The listing builds one solid part. Answer for the finished solid, in the listing's coordinates (mm). A direction names the side the tool comes from. Give positions to 0.01 mm unless a question says otherwise; leave off trailing zeros. Order: outer loops, then holes, each group sorted by start corner. A loop starts at its lowest first (then second) coordinate and runs counter-clockwise, first axis right, second up. Notation, with made-up numbers: (-28.75, 53.5) - (15.25, 53.5) arc R20 ccw to (15.25, 80.5) - close; hole circle Ø1 at (89.5, 65). An arc over 180 degrees is marked (long way). Use a Markdown table: item, result. Add a question column.
1) Flat-ended cylindrical pins translate along their axes: pin 1 (9 mm diameter, centred on x = -1, z = 0, fed in from +Y); pin 2 (5 mm diameter, centred on x = -12, z = 4.5, fed in from +Y); pin 3 (3 mm diameter, centred on y = -3.5, z = -6, fed in from -X). Find the tip coordinate at first contact, or state that the pin passes through.
2) For faces 4 (the face through (0, -8, 27.5)), 5 (the face through (0, -6, 21.5)), 6 (the face through (5, -4.6, 23.1)), 7 (the face through (0, -12, 25)), 8 (the face through (0, 4, -29.5)), determine the directions among +Z, -Z, +X, -X, +Y, -Y from which every point of the face is accessible in a straight line to the end or side of a thin tool.
3) The mould has two halves that part along Z. Classify faces 1 (the face through (-3.905, 2.986, -0.867)), 2 (the face through (0.07, -1.141, -8.703)), 3 (the face through (-16, 6, 0)): released by +Z, released by -Z, zero draft, split by the parting line, or undercut.
4) Find section B-B, the plane x = 0. State how many separate pieces and enclosed holes the cut face has, plus the area to 3 significant figures.
5) Straight lines are drawn through the part: line 1 (Y direction, x = -0.25, z = -4.5); line 2 (X direction, y = 4.5, z = 19.5); line 3 (Y direction, x = -9, z = -19). For each, find the intervals that lie inside material, in ascending order.
6) Find section D-D, the plane y = -9. Determine the outline of the cut face in (x, z).
7) Find section C-C, the plane z = 11.5. Determine the outline of the cut face in (x, y).
8) Find section A-A, the plane y = -6. Determine the outline of the cut face in (x, z), plus the area to 3 significant figures.
from build123d import *

# Parameters (mm, degrees)
SKETCH1_W           = 35
SKETCH1_H           = 63
BOSS_EXTRUDE1_DEPTH = 2
SKETCH2_W           = 10
SKETCH2_H           = 6
BOSS_EXTRUDE2_DEPTH = 12
SKETCH3_R           = 1.7
CUT_EXTRUDE1_DEPTH  = 10
FILLET1_R           = 4
SKETCH4_W           = 35
SKETCH4_H           = 63
SKETCH4_W_2         = 31
SKETCH4_H_2         = 59
BOSS_EXTRUDE4_DEPTH = 4
SKETCH5_R           = 4
BOSS_EXTRUDE5_DEPTH = 2


with BuildPart() as part:
    # Sketch1 → Boss-Extrude1 (new body)
    with BuildSketch(Plane(origin=(0, 0, 0), x_dir=(1, 0, 0), z_dir=(0, 1, 0))):
        Rectangle(SKETCH1_W, SKETCH1_H)
    extrude(amount=BOSS_EXTRUDE1_DEPTH)

    # Sketch2 → Boss-Extrude2 (add)
    with BuildSketch(Plane.XZ):
        with Locations((0, 24.5)):
            Rectangle(SKETCH2_W, SKETCH2_H)
        with Locations((0, -4.5)):
            Rectangle(SKETCH2_W, SKETCH2_H)
    extrude(amount=BOSS_EXTRUDE2_DEPTH)

    # Sketch3 → Cut-Extrude1 (cut)
    with BuildSketch(Plane(origin=(5, 0, 0), x_dir=(0, 0, -1), z_dir=(1, 0, 0))):
        with Locations((4.5, -6)):
            Circle(SKETCH3_R)
        with Locations((-24.5, -6)):
            Circle(SKETCH3_R)
    extrude(amount=-CUT_EXTRUDE1_DEPTH, mode=Mode.SUBTRACT)

    # Fillet1
    fillet1_edges = [part.edges().sort_by_distance(p)[0] for p in [
        (0, 0, 27.5),
        (0, 0, -7.5),
    ]]
    fillet(fillet1_edges, radius=FILLET1_R - 0.0001)  # a hair under: the kernel refuses the full size

    # Sketch4 → Boss-Extrude4 (add)
    with BuildSketch(Plane(origin=(0, 2, 0), x_dir=(1, 0, 0), z_dir=(0, 1, 0))):
        Rectangle(SKETCH4_W, SKETCH4_H)
        Rectangle(SKETCH4_W_2, SKETCH4_H_2, mode=Mode.SUBTRACT)
    extrude(amount=BOSS_EXTRUDE4_DEPTH)

    # Sketch5 → Boss-Extrude5 (add)
    with BuildSketch(Plane(origin=(0, 2, 0), x_dir=(1, 0, 0), z_dir=(0, 1, 0))):
        with Locations(Location((0, 0, 0), (0, 0, 270))):
            Circle(SKETCH5_R)
    extrude(amount=BOSS_EXTRUDE5_DEPTH)


solid = part.part
The answers:
| question | item | result |
|---|---|---|
| 1 | pin 1 | y = 4 |
| 1 | pin 2 | y = 2 |
| 1 | pin 3 | x = -5 |
| 2 | face 4 | +Z, +X, -X, -Y |
| 2 | face 5 | +X, -X, -Y |
| 2 | face 6 | +Z, -Z, +X, -Y |
| 2 | face 7 | +Z, -Z, +X, -X, -Y |
| 2 | face 8 | +Y |
| 3 | face 1 | undercut |
| 3 | face 2 | released by -Z |
| 3 | face 3 | zero draft |
| 4 | separate pieces | 1 |
| 4 | enclosed holes | 2 |
| 4 | area | 291 mm2 |
| 5 | line 1 | -12 to -7.7, -4.3 to 2 |
| 5 | line 2 | -17.5 to -15.5, 15.5 to 17.5 |
| 5 | line 3 | 0 to 2 |
| 6 | outline | (-5, -7.5) - (5, -7.5) - (5, -1.5) - (-5, -1.5) - close; (-5, 21.5) - (5, 21.5) - (5, 27.5) - (-5, 27.5) - close |
| 7 | outline | (-17.5, 0) - (17.5, 0) - (17.5, 6) - (15.5, 6) - (15.5, 2) - (-15.5, 2) - (-15.5, 6) - (-17.5, 6) - close |
| 8 | outline | (-5, -7.5) - (5, -7.5) - (5, -6.2) - (-5, -6.2) - close; (-5, -2.8) - (5, -2.8) - (5, -1.5) - (-5, -1.5) - close; (-5, 21.5) - (5, 21.5) - (5, 22.8) - (-5, 22.8) - close; (-5, 26.2) - (5, 26.2) - (5, 27.5) - (-5, 27.5) - close |
| 8 | area | 52.0 mm2 |
